Source: CAD feature listing. Evaluate the final solid. Frame: model axes, mm. A direction names the side the tool comes from. Round coordinates to 2 decimals unless told otherwise and drop trailing zeros. Loops run counter-clockwise (first coordinate to the right, second up) from the corner with the lowest first, then second, coordinate; pieces in that order, holes last. Notation, with made-up numbers: M -23.5,69 L 35.5,69 A13 cw 35.5,94 Z; hole C 41.5,47.25 d10. An arc over 180 degrees is marked long. Answer as a JSON object with one key per item and string values.
from build123d import *

# Parameters (mm, degrees)
RESSALTO_EXTRUS_O1_DEPTH = 8
ESBO_O2_R                = 1.5
CORTE_EXTRUS_O1_DEPTH    = 6
CHANFRO2_SIZE            = 1.5
FILETE1_R                = 2
FILETE2_R                = 1.5
FILETE3_R                = 0.65


with BuildPart() as part:
    # Esboço1 → Ressalto-extrusão1 (new body)
    with BuildSketch(Plane.XY):
        Polygon((-11.5, -1.2), (-11.5, 1.8), (-3.5, 1.8), (-3.5, 5), (22.5, 5), (22.5, 1.8), (30.5, 1.8), (30.5, -1.2), (19.5, -1.2), (19.5, 3), (4.5, 3), (4.5, 0.8), (-0.5, 0.8), (-0.5, -1.2), align=None)
    extrude(amount=RESSALTO_EXTRUS_O1_DEPTH)

    # Esboço2 → Corte-extrusão1 (cut)
    with BuildSketch(Plane(origin=(0, 1.8, 0), x_dir=(1, 0, 0), z_dir=(0, 1, 0))):
        with Locations(Location((-7.5, -4, 0), (0, 0, 180))):
            Circle(ESBO_O2_R)
        with Locations(Location((26.5, -4, 0), (0, 0, 180))):
            Circle(ESBO_O2_R)
    extrude(amount=-CORTE_EXTRUS_O1_DEPTH, mode=Mode.SUBTRACT)

    # Chanfro2
    chanfro2_edges = [part.edges().sort_by_distance(p)[0] for p in [
        (-6, 1.8, 4),
        (28, 1.8, 4),
    ]]
    chamfer(chanfro2_edges, length=CHANFRO2_SIZE)

    # Filete1
    filete1_edges = [part.edges().sort_by_distance(p)[0] for p in [
        (30.5, 0.3, 0),
        (-11.5, 0.3, 0),
        (-11.5, 0.3, 8),
        (-3.5, 5, 4),
        (22.5, 5, 4),
        (30.5, 0.3, 8),
    ]]
    fillet(filete1_edges, radius=FILETE1_R)

    # Filete2
    filete2_edges = [part.edges().sort_by_distance(p)[0] for p in [
        (19.5, 3, 4),
        (4.5, 3, 4),
    ]]
    fillet(filete2_edges, radius=FILETE2_R)

    # Filete3
    filete3_edges = [part.edges().sort_by_distance(p)[0] for p in [
        (12, 3, 0),
        (12, 3, 8),
        (19.5, 0.15, 0),
        (19.5, 0.15, 8),
        (4.939339828, 2.560660172, 0),
        (4.939339828, 2.560660172, 8),
        (19.060660172, 2.560660172, 0),
        (19.060660172, 2.560660172, 8),
        (4.5, 1.15, 0),
        (2, 0.8, 0),
        (-0.5, -0.2, 0),
        (-6.5, 1.8, 0),
        (22.5, 2.4, 0),
        (-6.5, 1.8, 8),
        (4.5, 0.8, 4),
        (-0.5, 0.8, 4),
        (-0.5, -0.2, 8),
        (2, 0.8, 8),
        (4.5, 1.15, 8),
        (30.5, 1.8, 4),
        (25.5, 1.8, 0),
        (25.5, 1.8, 8),
        (29.914213562, 1.8, 7.414213562),
        (29.914213562, 1.8, 0.585786438),
        (-3.5, 2.4, 0),
        (9.5, 5, 0),
        (-2.914213562, 4.414213562, 0),
        (21.914213562, 4.414213562, 0),
        (9.5, 5, 8),
        (-3.5, 2.4, 8),
        (-2.914213562, 4.414213562, 8),
        (21.914213562, 4.414213562, 8),
        (-11.5, 1.8, 4),
        (-10.914213562, 1.8, 7.414213562),
        (-10.914213562, 1.8, 0.585786438),
        (22.5, 2.4, 8),
    ]]
    fillet(filete3_edges, radius=FILETE3_R)


solid = part.part
Item 1: Section C-C on x = -4. Return the cut outline in (y, z), then the cut area to 3 significant figures.
Answer sheet:
{"outline": "M -1.2,0 L 1.15,0 A0.65 ccw 1.8,0.65 L 1.8,7.35 A0.65 ccw 1.15,8 L -1.2,8 Z", "area": "23.8 mm²"}
Item 2: Contact query for flat-ended pins moving along their axis: pin 1 Ø1.3 at (y, z) = (2.5, 3.5) entering from -X; pin 2 Ø3 at (x, z) = (2, 3) entering from -Y; pin 3 Ø2 at (x, z) = (-5.5, 3.5) entering from +Y. Output: stop coordinate, or through.
Answer sheet:
{"pin 1": "stops at x = -3.5", "pin 2": "stops at y = 0.8", "pin 3": "stops at y = 1.8"}
Item 3: Line query: probe 1 along Z at (x, y) = (-7.5, -0.65); probe 2 along X at (y, z) = (0, 3.25); probe 3 along Y at (x, z) = (8, 4). Output: solid intervals per line, ascending. Write a range as from..to.
Answer sheet:
{"probe 1": "z = 0..2.5, 5.5..8", "probe 2": "x = -11.5..-8.8, -6.2..-0.5, 19.5..25.2, 27.8..30.5", "probe 3": "y = 3..5"}
Item 4: Access query for faces 1 (the flat face through (-5, 1.8, 2)), 2 (the flat face through (19.5, 0, 4)), 3 (the flat face through (22.5, 2, 4)), 4 (the cylindrical face through (29.9, -0.04, 0.57)). Directions: +Z, -Z, +X, -X, +Y, -Y. A direction counts if a zero-diameter tool reaches every point of the face in a straight line with its end or side. Return the directions, or none.
Answer sheet:
{"face 1": "+Z, -Z, -X, +Y", "face 2": "+Z, -Z, -Y", "face 3": "+Z, -Z, +X, +Y", "face 4": "-Z, +X, +Y, -Y"}
Item 5: Section B-B on y = -0.5. Return the cut outline in (x, z), then the cut area to 3 significant figures.
Answer sheet:
{"outline": "M -11.5,2 A2 ccw -9.5,0 L -1.15,0 A0.65 ccw -0.5,0.65 L -0.5,7.35 A0.65 ccw -1.15,8 L -9.5,8 A2 ccw -11.5,6 Z; M 19.5,0.65 A0.65 ccw 20.15,0 L 28.5,0 A2 ccw 30.5,2 L 30.5,6 A2 ccw 28.5,8 L 20.15,8 A0.65 ccw 19.5,7.35 Z; hole C -7.5,4 d3; hole C 26.5,4 d3", "area": "158 mm²"}
Item 6: Pull-direction query (Z, two-part tool) for faces 5 (the cylindrical face through (-10.93, -0.01, 0.6)), 6 (the cylindrical face through (-10.93, -0.01, 7.4)), 7 (the flat face through (-11.5, 0, 4)), 8 (the cylindrical face through (-6, 0, 4)); classes: pulls with the +Z half, pulls with the -Z half, needs draft (parallel to the pull), parting line crosses it, or undercut.
Answer sheet:
{"face 5": "pulls with the -Z half", "face 6": "pulls with the +Z half", "face 7": "needs draft", "face 8": "undercut"}
Item 7: Section A-A on x = 26.5. Return the cut outline in (y, z).
Answer sheet:
{"outline": "M -1.2,0 L 1.15,0 A0.65 ccw 1.8,0.65 L 1.8,1 L 0.3,2.5 L -1.2,2.5 Z; M -1.2,5.5 L 0.3,5.5 L 1.8,7 L 1.8,7.35 A0.65 ccw 1.15,8 L -1.2,8 Z"}
